Input: part model. Units: mm. Frame: model coordinates. Face numbers are marked on the shaded views. A direction names the side the tool comes from. Coordinates: 2 decimals unless noted, no trailing zeros. Loops run counter-clockwise (first coordinate to the right, second up) from the corner with the lowest first, then second, coordinate; pieces in that order, holes last.
(1) Section A-A, the plane x = 0. Return loops of the section in (y, z), then the cut area to 3 significant figures.
(2) Section B-B, the plane y = 0. Return loops of the section in (x, z), then the cut area to 3 significant figures.
(3) Contact query for flat-ended pins moving along their axis: P1, Ø12, axis at y = -40, z = -32.5, coming from the +X side; P2, Ø2, axis at x = 25.5, y = 24.5, coming from the -Z side; P3, Ø5, axis at y = 1.5, z = -13.5, coming from the -X side. Output: stop coordinate, or through.
(4) Set-up query: the marked faces 1 and 2. Return all of +Z, -Z, +X, -X, +Y, -Y with unobstructed straight access to the full face (end or side cutting, diameter ignored); none if empty.
(5) Line query: L1, parallel to Y at x = 0.5, z = 64.5; L2, parallel to Y at x = -37.5, z = -15.5; L3, parallel to X at y = 30, z = 4.5. Output: solid intervals per line, ascending.
(6) Section D-D, the plane y = 17. Return loops of the section in (x, z).
(7) Section C-C, the plane z = 58. Return loops of the section in (x, y), then the cut area to 3 significant figures.
```python
from build123d import *

# Parameters (mm, degrees)
F2_R     = 10.504242
F3_DEPTH = 63.5
F4_R     = 2.216235


with BuildPart() as f1:
    # F0 (on Front) → F1 (revolve)
    with BuildSketch(Plane.XZ):
        with BuildLine():
            Line((0, -50.88574), (0, 50.88574))
            ThreePointArc((0, 50.88574), (-50.88574, 0), (0, -50.88574))
        make_face()
    revolve(axis=Axis((0, 0, 0), (0, 0, -1)))

    # F2 (on Top) → F3 (join)
    with BuildSketch(Plane.XY):
        Circle(F2_R)
    extrude(amount=F3_DEPTH)

    # F4 (on face) → F5 (revolve)
    with BuildSketch(Plane.XY.offset(63.5)):
        with Locations((0, 5.354275)):
            Circle(F4_R)
    revolve(axis=Axis((-0.112007, 0, 63.5), (1, 0, 0)))


solid = f1.part
```
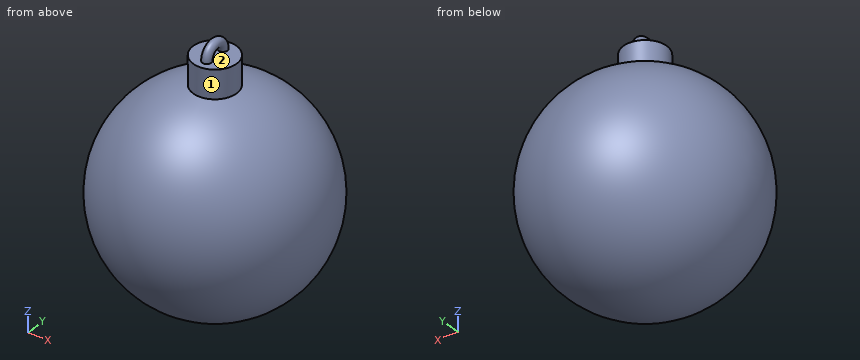
Report:
1. outline: (-10.5, 49.79) arc R50.89 ccw (long way) to (10.5, 49.79) - (10.5, 63.5) - (7.57, 63.5) arc R7.57 ccw to (-7.57, 63.5) - (-10.5, 63.5) - close; hole (-3.14, 63.5) - (3.14, 63.5) arc R3.14 ccw to start
1. area: 8,480 mm2
2. outline: (-10.5, 49.79) arc R50.89 ccw (long way) to (10.5, 49.79) - (10.5, 63.5) - (-10.5, 63.5) - close; circle Ø4.43 at (0, 68.85)
2. area: 8,420 mm2
3. P1: stops at x = 22.71
3. P2: stops at z = -37.53
3. P3: stops at x = -49.66
4. face 1: +Z
4. face 2: none
5. L1: y = -7.45 to -3.03, 3.03 to 7.45
5. L2: y = -30.71 to 30.71
5. L3: x = -40.85 to 40.85
6. outline: circle Ø95.92 at (0, 0)
7. outline: circle Ø21.01 at (0, 0)
7. area: 347 mm2
